from build123d import *

# Parameters (mm, degrees)
EXTRUDE_1_DEPTH     = 8
CUT_EXTRUDE_1_REACH = 28.93
SKETCH_3_W          = 2.2
SKETCH_3_H          = 4.2
CUT_EXTRUDE_2_REACH = 24.928
FILLET_1_R          = 1.5
FILLET_2_R          = 2
SKETCH_5_R          = 0.75
EXTRUDE_1_2_DEPTH   = 8


with BuildPart() as part:
    # 草图1 → Extrude 1 (new body)
    with BuildSketch(Plane(origin=(0, 0, 0), x_dir=(1, 0, 0), z_dir=(0, 1, 0))):
        with BuildLine():
            Line((-11, 9.5), (0, 9.5))
            ThreePointArc((0, 9.5), (6.646427612, 6.787856805), (9.497894504, 0.2))
            Line((9.497894504, 0.2), (12, 0.2))
            Line((12, 0.2), (12, -4.8))
            Line((12, -4.8), (14, -4.8))
            Line((14, -4.8), (14, 2.2))
            Line((14, 2.2), (11.28760382, 2.2))
            ThreePointArc((11.28760382, 2.2), (7.312660255, 8.875528153), (0, 11.5))
            Line((0, 11.5), (-11, 11.5))
            Line((-11, 11.5), (-11, 9.5))
        make_face()
    extrude(amount=EXTRUDE_1_DEPTH)

    # 草图3 → 切除-拉伸1 (cut, up to next)
    with BuildSketch(Plane.ZY.offset(-12), mode=Mode.PRIVATE) as cut_extrude_1_sk1:
        with Locations((0.9, 4)):
            Rectangle(SKETCH_3_W, SKETCH_3_H)
    cut_extrude_1_tool1 = extrude(cut_extrude_1_sk1.sketch, amount=-CUT_EXTRUDE_1_REACH, mode=Mode.PRIVATE) & part.part
    add(cut_extrude_1_tool1.solids().sort_by_distance((12, 4, 0.9))[0], mode=Mode.SUBTRACT)

    # 草图4 → 切除-拉伸2 (cut, up to next)
    with BuildSketch(Plane(origin=(0, 0, -11.5), x_dir=(-1, 0, 0), z_dir=(0, 0, -1)), mode=Mode.PRIVATE) as cut_extrude_2_sk1:
        with BuildLine():
            Line((11, 2.4), (8.5, 2.4))
            ThreePointArc((8.5, 2.4), (6.9, 4), (8.5, 5.6))
            Line((8.5, 5.6), (11, 5.6))
            ThreePointArc((11, 5.6), (12.6, 4), (11, 2.4))
        make_face()
    cut_extrude_2_tool1 = extrude(cut_extrude_2_sk1.sketch, amount=-CUT_EXTRUDE_2_REACH, mode=Mode.PRIVATE) & part.part
    add(cut_extrude_2_tool1.solids().sort_by_distance((-9.75, 4, -11.5))[0], mode=Mode.SUBTRACT)

    # 圆角1
    fillet_1_edges = [part.edges().sort_by_distance(p)[0] for p in [
        (11.28760382, 4, -2.2),
        (14, 4, -2.2),
        (9.497894504, 4, -0.2),
    ]]
    fillet(fillet_1_edges, radius=FILLET_1_R)

    # 圆角2
    fillet_2_edges = [part.edges().sort_by_distance(p)[0] for p in [
        (13, 8, 4.8),
        (13, 0, 4.8),
    ]]
    fillet(fillet_2_edges, radius=FILLET_2_R)

    # 草图5 → Extrude 1 2 (add)
    with BuildSketch(Plane(origin=(0, 8, 0), x_dir=(1, 0, 0), z_dir=(0, 1, 0))):
        with Locations((-2, 9.5)):
            Circle(SKETCH_5_R)
    extrude(amount=-EXTRUDE_1_2_DEPTH)


solid = part.part
Verification items for the finished model (mm, model axes). A direction names the side the tool comes from. Coordinates: 2 decimals unless noted, no trailing zeros. Loops run counter-clockwise (first coordinate to the right, second up) from the corner with the lowest first, then second, coordinate; pieces in that order, holes last. Notation, with made-up numbers: (20, -18.5) -> (34, -18.5) arc R25 ccw to (34, 8.5) -> close; hole circle Ø5 at (45.25, 74.5). An arc over 180 degrees is marked (long way). Answer as CSV lines item,"result".
1) Release check for a two-part mould opening along Z. For faces 5 (the cylindrical face through (6.105, 3.944, -7.279)), 6 (the flat face through (3.3, 0, -9.2)), 7 (the flat face through (13, 4, 2)) record: +Z half, -Z half, draft (parallel to the pull), parting line (faces both ways), or undercut.
Found:
face 5,"+Z half"
face 6,"draft"
face 7,"undercut"
2) Thickness scan on L1, parallel to X at y = 2.25, z = 2.75; L2, parallel to Z at x = -7.5, y = 1.25; L3, parallel to Z at x = 12.75, y = 2.5. Record the ranges inside material, lowest first. Write a range as from..to.
Found:
L1,"x = 12..14"
L2,"z = -11.5..-9.5"
L3,"z = -2.18..-0.2, 2..4.8"
3) Depth check by flat-ended pin: pin 1 (2.5 mm diameter, centred on y = 4, z = 1.5, fed in from -X); pin 2 (2 mm diameter, centred on y = 6.5, z = -7.5, fed in from +X); pin 3 (1 mm diameter, centred on y = 1, z = -6, fed in from -X). Enter the tip coordinate at first touch or a pass-through.
Found:
pin 1,"stops at x = 12"
pin 2,"stops at x = 9.49"
pin 3,"stops at x = 6.93"
4) Tool access check on faces 1 (the flat face through (13, 1.9, 1)), 2 (the flat face through (-10, 2.4, -11)), 3 (the flat face through (-6, 4, -9.5)), 4 (the flat face through (-11, 1, -11)). Record the directions out of +Z, -Z, +X, -X, +Y, -Y that give a thin tool (end or side, any length) a straight path to the whole face; none if there is none.
Found:
face 1,"+X, -X"
face 2,"+Z, -Z, -X"
face 3,"+Z, -X, +Y, -Y"
face 4,"+Z, -Z, -X, +Y, -Y"
5) Cross-section at D-D, the plane z = -8. Record the cut outline in (x, y), then the cut area to 3 significant figures.
Found:
outline,"(5.12, 0) -> (8.26, 0) -> (8.26, 8) -> (5.12, 8) -> close"
area,"25.1 mm2"
6) Cross-section at C-C, the plane x = -0.25. Record the cut outline in (y, z), then the cut area to 3 significant figures.
Found:
outline,"(0, -11.5) -> (8, -11.5) -> (8, -9.5) -> (0, -9.5) -> close"
area,"16.0 mm2"
